Could you check a few things on this model? Use its own coordinates, in mm. Face numbers are marked on the shaded views. A direction names the side the tool comes from. Give positions to 0.01 mm unless a question says otherwise; leave off trailing zeros. Write each loop counter-clockwise with the first axis right and the second up, starting at its lowest first coordinate (ties: lowest second). Pieces come first, ordered by that corner, then holes. Notation, with made-up numbers: (3.5, -14.5) - (39.5, -14.5) arc R23 cw to (39.5, -6.5) - close; hole circle Ø3 at (66, 18.5). An arc over 180 degrees is marked (long way). Use one line per item in the form item = value.
```python
from build123d import *

# Parameters (mm, degrees)
SKETCH1_R               = 1.85
BOSS_EXTRUDE1_DEPTH     = 3
SKETCH2_W               = 3
SKETCH2_H               = 48
BOSS_EXTRUDE2_DEPTH     = 26.75
SKETCH4_W               = 24
SKETCH4_H               = 16.5
SKETCH4_R               = 0.9
CUT_EXTRUDE3_DEPTH      = 3
CUT_EXTRUDE4_DEPTH      = 92.395308961
CUT_EXTRUDE4_DEPTH_BACK = 3
SKETCH6_W               = 3
SKETCH6_H               = 15
BOSS_EXTRUDE3_DEPTH     = 26.75
CUT_EXTRUDE5_DEPTH      = 6
SKETCH8_R               = 2.1
CUT_EXTRUDE6_DEPTH      = 6
FILLET2_R               = 3
SKETCH10_R              = 4
SKETCH10_R_2            = 1.85
BOSS_EXTRUDE4_DEPTH     = 3


with BuildPart() as part:
    # Sketch1 → Boss-Extrude1 (new body)
    with BuildSketch(Plane(origin=(0, 0, 0), x_dir=(1, 0, 0), z_dir=(0, 1, 0))):
        with BuildLine():
            Line((52, 55.2), (52, 50))
            Line((52, 50), (37, 50))
            Line((37, 50), (37, 42.5))
            Line((37, 42.5), (19.85, 42.5))
            Line((19.85, 42.5), (19.85, 30))
            Line((19.85, 30), (0, 30))
            Line((0, 30), (0, 0))
            Line((0, 0), (62, 0))
            Line((62, 0), (62, 50))
            Line((62, 50), (62, 55.2))
            ThreePointArc((62, 55.2), (57, 60.2), (52, 55.2))
        make_face()
        with Locations(Location((31, 25, 0), (0, 0, 270))):
            Circle(SKETCH1_R, mode=Mode.SUBTRACT)
        with Locations(Location((57, 55.2, 0), (0, 0, 270))):
            Circle(SKETCH1_R, mode=Mode.SUBTRACT)
    extrude(amount=-BOSS_EXTRUDE1_DEPTH)

    # Sketch2 → Boss-Extrude2 (add)
    with BuildSketch(Plane(origin=(0, -3, 0), x_dir=(-1, 0, 0), z_dir=(0, -1, 0))):
        with Locations((-60.5, 24)):
            Rectangle(SKETCH2_W, SKETCH2_H)
        with Locations((-1.5, 24)):
            Rectangle(SKETCH2_W, SKETCH2_H)
    extrude(amount=BOSS_EXTRUDE2_DEPTH)

    # Sketch4 → Cut-Extrude3 (cut)
    with BuildSketch(Plane.ZY.offset(-62)):
        with BuildLine():
            Line((-48, -29.75), (-34.625, -29.75))
            ThreePointArc((-34.625, -29.75), (-43.69937868, -25.44937868), (-48, -16.375))
            Line((-48, -16.375), (-48, -29.75))
        make_face()
        with Locations((-19.65, -21.5)):
            Rectangle(SKETCH4_W, SKETCH4_H)
        with BuildLine():
            ThreePointArc((0, -22.1), (-2.240633124, -27.509366876), (-7.65, -29.75))
            Line((-7.65, -29.75), (0, -29.75))
            Line((0, -29.75), (0, -22.1))
        make_face()
        with Locations((-33.5, -21.5)):
            Circle(SKETCH4_R)
        with Locations(Location((-5.8, -21.5, 0), (0, 0, 180))):
            Circle(SKETCH4_R)
    cut_extrude3 = extrude(amount=CUT_EXTRUDE3_DEPTH, mode=Mode.SUBTRACT)

    # Mirror2: Cut-Extrude3 across plane
    add(cut_extrude3.mirror(Plane(origin=(31, 0, 0), x_dir=(0, 0, 1), z_dir=(1, 0, 0))), mode=Mode.SUBTRACT)

    # Sketch5 → Cut-Extrude4 (cut, two sides: drawn at the far end of the back side and taken through both)
    with BuildSketch(Plane.ZY.offset(-CUT_EXTRUDE4_DEPTH_BACK)):
        with BuildLine():
            Line((-48, -3), (-48, -16.375))
            ThreePointArc((-48, -16.375), (-43.861015127, -7.138984873), (-34.625, -3))
            Line((-34.625, -3), (-48, -3))
        make_face()
    extrude(amount=CUT_EXTRUDE4_DEPTH + CUT_EXTRUDE4_DEPTH_BACK, mode=Mode.SUBTRACT)

    # Sketch6 → Boss-Extrude3 (add)
    with BuildSketch(Plane(origin=(0, -3, 0), x_dir=(-1, 0, 0), z_dir=(0, -1, 0))):
        with Locations((-34, 33.899748742)):
            Rectangle(SKETCH6_W, SKETCH6_H)
        with Locations((-34, 14)):
            Rectangle(SKETCH6_W, SKETCH6_H)
    extrude(amount=BOSS_EXTRUDE3_DEPTH)

    # Sketch7 → Cut-Extrude5 (cut)
    with BuildSketch(Plane.ZY.offset(-32.5)):
        with BuildLine():
            Line((-6.5, -29.75), (-6.5, -21.5))
            ThreePointArc((-6.5, -21.5), (-14, -29), (-21.5, -21.5))
            Line((-21.5, -21.5), (-21.5, -29.75))
            Line((-21.5, -29.75), (-6.5, -29.75))
        make_face()
        with BuildLine():
            ThreePointArc((-16.1, -21.5), (-14, -23.6), (-11.9, -21.5))
            Line((-11.9, -21.5), (-16.1, -21.5))
        make_face()
        with BuildLine():
            Line((-16.1, -21.5), (-11.9, -21.5))
            ThreePointArc((-11.9, -21.5), (-14, -19.4), (-16.1, -21.5))
        make_face()
    extrude(amount=-CUT_EXTRUDE5_DEPTH, mode=Mode.SUBTRACT)

    # Sketch8 → Cut-Extrude6 (cut)
    with BuildSketch(Plane.ZY.offset(-32.5)):
        with Locations((-33.899748742, -21.5)):
            Circle(SKETCH8_R)
        with BuildLine():
            ThreePointArc((-26.399748742, -21.5), (-33.899748742, -29), (-41.399748742, -21.5))
            Line((-41.399748742, -21.5), (-41.399748742, -29.75))
            Line((-41.399748742, -29.75), (-26.399748742, -29.75))
            Line((-26.399748742, -29.75), (-26.399748742, -21.5))
        make_face()
    extrude(amount=-CUT_EXTRUDE6_DEPTH, mode=Mode.SUBTRACT)

    # Fillet2
    fillet2_edges = [part.edges().sort_by_distance(p)[0] for p in [
        (19.85, -1.5, -42.5),
        (37, -1.5, -50),
    ]]
    fillet(fillet2_edges, radius=FILLET2_R)

    # Sketch10 → Boss-Extrude4 (add)
    with BuildSketch(Plane.XZ.offset(3)):
        with Locations(Location((57, -55.2, 0), (0, 0, 90))):
            Circle(SKETCH10_R)
        with Locations(Location((57, -55.2, 0), (0, 0, 90))):
            Circle(SKETCH10_R_2, mode=Mode.SUBTRACT)
    extrude(amount=BOSS_EXTRUDE4_DEPTH)


solid = part.part
```
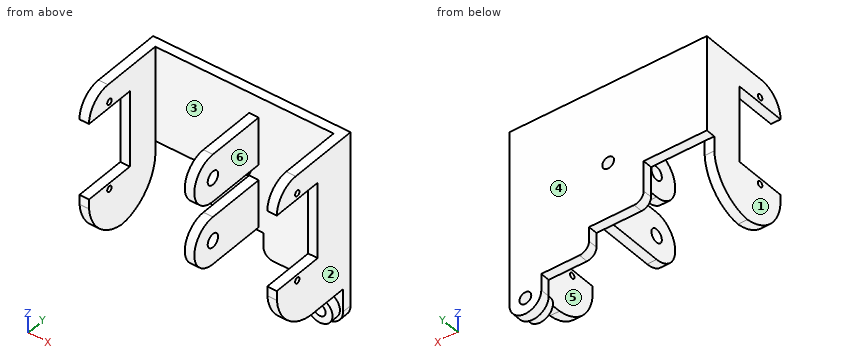
1. Imagine slicing it at B-B, the plane z = -45.5. List the corners of the cut face in (x, y) for me.
Response values:
outline = (0, -23.27) - (3, -23.27) - (3, -9.1) - (0, -9.1) - close; (37, -3) - (59, -3) - (59, -23.27) - (62, -23.27) - (62, 0) - (37, 0) - close
2. Which directions (+Z, -Z, +X, -X, +Y, -Y) give clear straight access to the entire face, cutting with the end or side of a thin tool? Please do the marked faces 4, 5 and 6.
Response values:
face_4 = +Z, -Z, +X, -X, +Y
face_5 = +Z, -Y
face_6 = +Z, -Z, -Y
3. Imagine slicing it at A-A, the plane x = 31. List the corners of the cut face in (y, z) for me.
Response values:
outline = (-3, -42.5) - (0, -42.5) - (0, -26.85) - (-3, -26.85) - close; (-3, -23.15) - (0, -23.15) - (0, 0) - (-3, 0) - close
4. Imagine slicing it at D-D, the plane z = -18.5. List the corners of the cut face in (x, y) for me, and give its area (3 significant figures).
Response values:
outline = (0, -13.25) - (3, -13.25) - (3, -3) - (32.5, -3) - (32.5, -27.5) - (35.5, -27.5) - (35.5, -3) - (59, -3) - (59, -13.25) - (62, -13.25) - (62, 0) - (0, 0) - close
area = 321 mm²
5. For pin 1 (5 mm diameter, centred on x = 41, z = -37, fed in from -Y); pin 2 (8 mm diameter, centred on y = -4, z = -44.5, fed in from -X); pin 3 (5 mm diameter, centred on x = 57, z = -55.2, fed in from -Y); pin 4 (10 mm diameter, centred on y = -26, z = -13, fed in from -X), each with a flat end and sliding along its axis, tell me the tip position at first contact or that it passes through.
Response values:
pin_1 = -3
pin_2 = 0
pin_3 = -6
pin_4 = 32.5
6. Imagine slicing it at C-C, the plane y = -9. List the corners of the cut face in (x, z) for me, and give its area (3 significant figures).
Response values:
outline = (0, -45.43) - (3, -45.43) - (3, 0) - (0, 0) - close; (32.5, -41.4) - (35.5, -41.4) - (35.5, -26.4) - (32.5, -26.4) - close; (32.5, -21.5) - (35.5, -21.5) - (35.5, -6.5) - (32.5, -6.5) - close; (59, -48) - (62, -48) - (62, 0) - (59, 0) - close
area = 370 mm²
7. If we mould it in two halves opening along X, with no side actions, what happens to the marked faces 1, 2 and 3? For each: pulls with the +X half, pulls with the -X half, needs draft (parallel to the pull), parting line crosses it, or undercut.
Response values:
face_1 = pulls with the -X half
face_2 = pulls with the +X half
face_3 = undercut
8. If I drill on line 1 (X direction, y = -23.5, z = -39.5); line 2 (Z direction, x = 34, y = -8.75); line 3 (X direction, y = -1.3, z = -25), over which ranges is the centre line in solid material (lowest first)? Write a range as from..to.
Response values:
line_1 = 0..3, 32.5..35.5, 59..62
line_2 = -41.4..-26.4, -21.5..-6.5
line_3 = 0..29.15, 32.85..62
